from build123d import *

# Parameters (mm, degrees)
SKETCH_1_W          = 32
SKETCH_1_H          = 13
EXTRUDE_1_DEPTH     = 3
SKETCH_2_R          = 1.75
CUT_EXTRUDE_1_DEPTH = 4
EXTRUDE_2_DEPTH     = 3


with BuildPart() as part:
    # 스케치1 → 보스-돌출1 (new body)
    with BuildSketch(Plane(origin=(0, 0, 0), x_dir=(1, 0, 0), z_dir=(0, 1, 0))):
        Rectangle(SKETCH_1_W, SKETCH_1_H)
    extrude(amount=EXTRUDE_1_DEPTH)

    # 스케치2 → 컷-돌출1 (cut, through all)
    with BuildSketch(Plane(origin=(0, 3, 0), x_dir=(1, 0, 0), z_dir=(0, 1, 0))):
        with Locations((-12.5, -4)):
            Circle(SKETCH_2_R)
        with Locations((12.5, -4)):
            Circle(SKETCH_2_R)
    extrude(amount=-CUT_EXTRUDE_1_DEPTH, mode=Mode.SUBTRACT)

    # 스케치3 → 보스-돌출2 (add)
    with BuildSketch(Plane.XZ):
        Polygon((-8.75, 6.5), (8.75, 6.5), (8.75, -3.5), (16, -3.5), (16, -6.5), (-16, -6.5), (-16, -3.5), (-8.75, -3.5), align=None)
    extrude(amount=EXTRUDE_2_DEPTH)


solid = part.part
Check sheet for the modelled part. Datum: model origin and axes. Units: mm. A direction names the side the tool comes from. Round coordinates to 2 decimals unless told otherwise and drop trailing zeros. Loops run counter-clockwise (first coordinate to the right, second up) from the corner with the lowest first, then second, coordinate; pieces in that order, holes last.
1. Scan lines: probe 1 along X at (y, z) = (1.6, 4); probe 2 along Z at (x, y) = (-12.5, 2.2); probe 3 along X at (y, z) = (1.2, 5). Record each from-to range of solid material in increasing order.
2. Sectioned sample at A-A on z = 4. Record the boundary of the cut face in (x, y), and give its area (4 significant figures).
3. Set-up check for faces 5 (the flat face through (-12, -1, -3.5)), 6 (the flat face through (8.75, -1, 2)), 7 (the flat face through (0, 1, 6.5)): record each of +Z, -Z, +X, -X, +Y, -Y from which the full face is reachable in a straight line by a thin tool's end or side.
4. Sectioned sample at C-C on y = 1.4. Record the boundary of the cut face in (x, z), and give its area (3 significant figures).
5. Sectioned sample at D-D on z = 1.5. Record the boundary of the cut face in (x, y), and give its area (4 significant figures).
6. Sectioned sample at B-B on x = -12.5. Record the boundary of the cut face in (y, z), and give its area (3 significant figures).
7. Mould release check, pull along X, two halves, no side actions. Record for faces 1 (the flat face through (-12, 0, 1)), 2 (the flat face through (16, 1, -1)), 3 (the cylindrical face through (-10.883, 1.521, 4.67)), 4 (the flat face through (-16, 1, -1)): released by +X, released by -X, zero draft, split by the parting line, or undercut.
8. Gauge pin test, flat ends, axial feed: pin 1 Ø2.5 at (y, z) = (-2, 3.5) entering from +X; pin 2 Ø0.9 at (x, y) = (-11, -1) entering from +Z; pin 3 Ø3 at (x, z) = (-12.5, 4) entering from +Y; pin 4 Ø2.5 at (y, z) = (-2, 0.5) entering from -X. Record the tip position at first contact, or that the pin passes through.
Recorded:
1. probe 1: x = -16 to -14.25, -10.75 to 10.75, 14.25 to 16
1. probe 2: z = -6.5 to 2.25, 5.75 to 6.5
1. probe 3: x = -16 to -13.94, -11.06 to 11.06, 13.94 to 16
2. outline: (-16, 0) - (-14.25, 0) - (-14.25, 3) - (-16, 3) - close; (-10.75, 0) - (-8.75, 0) - (-8.75, -3) - (8.75, -3) - (8.75, 0) - (10.75, 0) - (10.75, 3) - (-10.75, 3) - close; (14.25, 0) - (16, 0) - (16, 3) - (14.25, 3) - close
2. area: 127.5 mm2
3. face 5: +Z, -X, -Y
3. face 6: +Z, +X, -Y
3. face 7: +Z, +X, -X, +Y, -Y
4. outline: (-16, -6.5) - (16, -6.5) - (16, 6.5) - (-16, 6.5) - close; hole circle Ø3.5 at (-12.5, 4); hole circle Ø3.5 at (12.5, 4)
4. area: 397 mm2
5. outline: (-16, 0) - (-8.75, 0) - (-8.75, -3) - (8.75, -3) - (8.75, 0) - (16, 0) - (16, 3) - (-16, 3) - close
5. area: 148.5 mm2
6. outline: (-3, -6.5) - (3, -6.5) - (3, 2.25) - (0, 2.25) - (0, -3.5) - (-3, -3.5) - close; (0, 5.75) - (3, 5.75) - (3, 6.5) - (0, 6.5) - close
6. area: 37.5 mm2
7. face 1: zero draft
7. face 2: released by +X
7. face 3: undercut
7. face 4: released by -X
8. pin 1: stops at x = 8.75
8. pin 2: stops at z = -3.5
8. pin 3: passes through
8. pin 4: stops at x = -8.75
